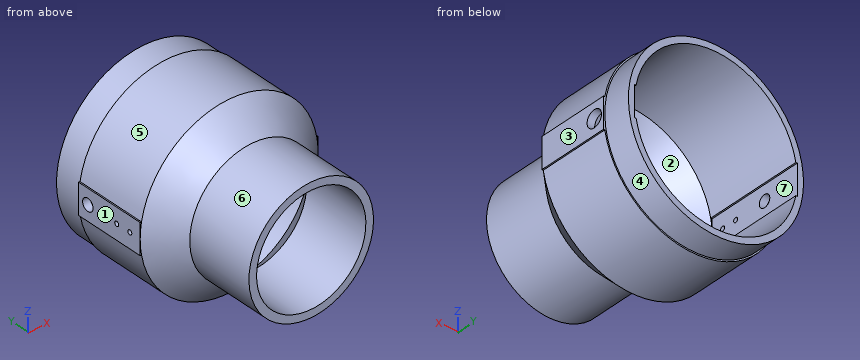
```python
from build123d import *

# Parameters (mm, degrees)
SKETCH14_W              = 0.91
SKETCH14_H              = 18
SKETCH8_W               = 20
SKETCH8_H               = 47
BOSS_EXTRUDE1_DEPTH     = 0.862384063
CUT_EXTRUDE4_REACH      = 181.492
CUT_EXTRUDE4_END_RADIUS = 53.41
SKETCH10_W              = 20
SKETCH10_H              = 65
CIRPATTERN1_COUNT       = 2
SKETCH11_R              = 5.5
CUT_EXTRUDE5_DEPTH      = 5
SKETCH12_R              = 4
SKETCH12_R_2            = 1.515
CUT_EXTRUDE6_DEPTH      = 5


with BuildPart() as part:
    # Sketch1 → Revolve1 (revolve)
    with BuildSketch(Plane.XY, mode=Mode.PRIVATE) as revolve1_sk:
        Polygon((58.41, -65), (40.91, -82.5), (40.91, -127.679491924), (35.91, -127.679491924), (35.91, -82.5), (53.41, -65), (53.41, 0), (58.41, 0), align=None)
    revolve(revolve1_sk.sketch.rotate(Axis((0, 0, 0), (0, -1, 0)), 90), axis=Axis((0, 0, 0), (0, -1, 0)))

    # Sketch14 → Cut-Revolve5 (revolve, cut)
    with BuildSketch(Plane.XY, mode=Mode.PRIVATE) as cut_revolve5_sk:
        with Locations((-57.955, -9)):
            Rectangle(SKETCH14_W, SKETCH14_H)
    revolve(cut_revolve5_sk.sketch.rotate(Axis((0, 0, 0), (0, 1, 0)), 90), axis=Axis((0, 0, 0), (0, 1, 0)), mode=Mode.SUBTRACT)

    # Sketch8 → Boss-Extrude1 (add)
    with BuildSketch(Plane.ZY.offset(58.41)):
        with Locations((0, -41.5)):
            Rectangle(SKETCH8_W, SKETCH8_H)
    boss_extrude1 = extrude(amount=-BOSS_EXTRUDE1_DEPTH)

    # Cut-Extrude4: up to this cylinder (the profile starts outside it)
    cut_extrude4_end = Plane(origin=(0, -32.5, 0), z_dir=(0, 1, 0)) * Cylinder(CUT_EXTRUDE4_END_RADIUS, 470.804, mode=Mode.PRIVATE)
    # Sketch10 → Cut-Extrude4 (cut, up to the surface)
    with BuildSketch(Plane(origin=(-53.41, 0, 0), x_dir=(0, 0, -1), z_dir=(1, 0, 0)), mode=Mode.PRIVATE) as cut_extrude4_sk1:
        with Locations((0, -32.5)):
            Rectangle(SKETCH10_W, SKETCH10_H)
    cut_extrude4_tool1 = extrude(cut_extrude4_sk1.sketch, amount=CUT_EXTRUDE4_REACH, mode=Mode.PRIVATE) - cut_extrude4_end
    cut_extrude4 = cut_extrude4_tool1.solids().sort_by_distance((-53.41, -32.5, 0))[0] + cut_extrude4_tool1.solids().sort_by_distance((-53.41, -32.5, 0))[1]
    add(cut_extrude4, mode=Mode.SUBTRACT)

    # CirPattern1: Boss-Extrude1, Cut-Extrude4 ×2 about axis
    cirpattern1_axis = Axis((0, 0, 0), (0, 1, 0))
    add([boss_extrude1.rotate(cirpattern1_axis, i * 360 / CIRPATTERN1_COUNT) for i in range(1, CIRPATTERN1_COUNT)])
    add([cut_extrude4.rotate(cirpattern1_axis, i * 360 / CIRPATTERN1_COUNT) for i in range(1, CIRPATTERN1_COUNT)], mode=Mode.SUBTRACT)

    # Sketch11 → Cut-Extrude5 (cut)
    with BuildSketch(Plane(origin=(58.41, 0, 0), x_dir=(0, 0, -1), z_dir=(1, 0, 0))):
        with Locations((0, -25)):
            Circle(SKETCH11_R)
    extrude(amount=-CUT_EXTRUDE5_DEPTH, mode=Mode.SUBTRACT)

    # Sketch12 → Cut-Extrude6 (cut)
    with BuildSketch(Plane.ZY.offset(58.41)):
        with Locations((0, -25)):
            Circle(SKETCH12_R)
        with Locations((0, -47.0538)):
            Circle(SKETCH12_R_2)
        with Locations((0, -57.0538)):
            Circle(SKETCH12_R_2)
    extrude(amount=-CUT_EXTRUDE6_DEPTH, mode=Mode.SUBTRACT)


solid = part.part
```
The listing builds one solid part. Answer for the finished solid, in the listing's coordinates (mm). Face numbers are marked on the shaded views. A direction names the side the tool comes from. Give positions to 0.01 mm unless a question says otherwise; leave off trailing zeros. Write each loop counter-clockwise with the first axis right and the second up, starting at its lowest first coordinate (ties: lowest second). Pieces come first, ordered by that corner, then holes. Notation, with made-up numbers: (-1.75, -17.5) - (29.25, -17.5) arc R28 cw to (29.25, 8.5) - close; hole circle Ø10 at (-8, -40). An arc over 180 degrees is marked (long way). Use one line per item in the form item = value. Start each with the question number.
1) Find section A-A on x = 0. Determine the outline of the cut face in (y, z), plus the area to 3 significant figures.
2) Find section C-C on y = -94.5. Determine the outline of the cut face in (x, z).
3) A tool of negligible diameter and unlimited length cuts with its end or side. For the marked faces 5, 6 and 7, from which of +Z, -Z, +X, -X, +Y, -Y can it reach the whole face along a straight path? Write none if from no direction.
4) Find section B-B on y = -25. Determine the outline of the cut face in (x, z), plus the area to 3 significant figures.
5) Flat-ended cylindrical pins translate along their axes: pin 1 Ø6 at (y, z) = (-86.5, 39) entering from -X; pin 2 Ø12 at (x, y) = (31.5, -63) entering from -Z; pin 3 Ø0.7 at (x, z) = (58, -3) entering from -Y. Find the tip coordinate at first contact, or state that the pin passes through.
6) Consider line 1 along X through (y, z) = (-99.5, 0); line 2 along Z through (x, y) = (-1.5, -31); line 3 along Z through (x, y) = (10, -47.5). Determine where each line is inside the solid, lowest interval first. Write a range as from..to.
7) The mould has two halves that part along X. Classify the marked faces 1, 2, 3 and 4: pulls with the +X half, pulls with the -X half, needs draft (parallel to the pull), parting line crosses it, or undercut.
Geometry results:
q1.outline = (-127.68, -40.91) - (-82.5, -40.91) - (-65, -58.41) - (-18, -58.41) - (-18, -57.5) - (0, -57.5) - (0, -53.41) - (-65, -53.41) - (-82.5, -35.91) - (-127.68, -35.91) - close; (-127.68, 35.91) - (-82.5, 35.91) - (-65, 53.41) - (0, 53.41) - (0, 57.5) - (-18, 57.5) - (-18, 58.41) - (-65, 58.41) - (-82.5, 40.91) - (-127.68, 40.91) - close
q1.area = 1,240 mm2
q2.outline = circle Ø81.82 at (0, 0); hole circle Ø71.82 at (0, 0)
q3.face_5 = +Z, +Y, -Y
q3.face_6 = -Y
q3.face_7 = +Y
q4.outline = (-58.41, -10) - (-57.55, -10) arc R58.41 ccw to (57.55, -10) - (58.41, -10) - (58.41, -5.5) - (53.41, -5.5) - (53.41, -10) - (52.47, -10) arc R53.41 cw to (-52.47, -10) - (-53.41, -10) - (-53.41, -4) - (-58.41, -4) - close; (-58.41, 4) - (-53.41, 4) - (-53.41, 10) - (-52.47, 10) arc R53.41 cw to (52.47, 10) - (53.41, 10) - (53.41, 5.5) - (58.41, 5.5) - (58.41, 10) - (57.55, 10) arc R58.41 ccw to (-57.55, 10) - (-58.41, 10) - close
q4.area = 1,660 mm2
q5.pin_1 = -19.43
q5.pin_2 = -52.55
q5.pin_3 = -65.68
q6.line_1 = -40.91..-35.91, 35.91..40.91
q6.line_2 = -58.39..-53.39, 53.39..58.39
q6.line_3 = -57.55..-52.47, 52.47..57.55
q7.face_1 = pulls with the -X half
q7.face_2 = undercut
q7.face_3 = pulls with the +X half
q7.face_4 = parting line crosses it
